```python
from build123d import *

# Parameters (mm, degrees)
ESQUISSE1_W             = 68
ESQUISSE1_H             = 1.6
EXTRUSION1_DEPTH        = 45
ESQUISSE2_W             = 25
ESQUISSE2_H             = 34
ENL_V_MAT_EXTRU_1_DEPTH = 2
ESQUISSE4_W             = 4.000005344
ESQUISSE4_H             = 8.5
ENL_V_MAT_EXTRU_2_DEPTH = 0.1
ESQUISSE5_W             = 4.000005344
ESQUISSE5_H             = 8.5
ENL_V_MAT_EXTRU_3_DEPTH = 0.1


with BuildPart() as part:
    # Esquisse1 → Extrusion1 (new body)
    with BuildSketch(Plane.XY):
        with Locations((57.011095297, 71.602293989)):
            Rectangle(ESQUISSE1_W, ESQUISSE1_H)
    extrude(amount=EXTRUSION1_DEPTH)

    # Esquisse2 → Enlèv. mat.-Extru.1 (cut)
    with BuildSketch(Plane(origin=(0, 72.402293989, 0), x_dir=(-1, 0, 0), z_dir=(0, 1, 0))):
        with Locations((-78.511095297, 47)):
            Rectangle(ESQUISSE2_W, ESQUISSE2_H)
    extrude(amount=-ENL_V_MAT_EXTRU_1_DEPTH, mode=Mode.SUBTRACT)

    # Esquisse4 → Enlèv. mat.-Extru.2 (cut)
    with BuildSketch(Plane(origin=(0, 72.402293989, 0), x_dir=(-1, 0, 0), z_dir=(0, 1, 0))):
        with Locations((-89.011092625, 4.25)):
            Rectangle(ESQUISSE4_W, ESQUISSE4_H)
        Polygon((-27.011089953, 8.5), (-27.011089953, 0), (-23.011095297, 0), (-23.029811449, 8.5), align=None)
        Polygon((-83.761089902, 23.952607164), (-71.261089902, 23.952607164), (-71.261089902, 29.947835896), (-83.761089902, 30.082433695), align=None)
    extrude(amount=-ENL_V_MAT_EXTRU_2_DEPTH, mode=Mode.SUBTRACT)

    # Esquisse5 → Enlèv. mat.-Extru.3 (cut)
    with BuildSketch(Plane.XZ.offset(-70.802293989)):
        Polygon((23.029811449, 8.5), (23.011095297, 0), (27.011089953, 0), (27.011089953, 8.5), align=None)
        with Locations((89.011092625, 4.25)):
            Rectangle(ESQUISSE5_W, ESQUISSE5_H)
    extrude(amount=-ENL_V_MAT_EXTRU_3_DEPTH, mode=Mode.SUBTRACT)


solid = part.part
```
Here's how the part is built. I have some questions about the finished solid (model axes, mm). A direction names the side the tool comes from. Round coordinates to 2 decimals unless told otherwise and drop trailing zeros. Write each loop counter-clockwise with the first axis right and the second up, starting at its lowest first coordinate (ties: lowest second). Pieces come first, ordered by that corner, then holes.
Q1. If we mould it in two halves opening along Z, with no side actions, what happens to faces 6 (the flat face through (78, 72.302, 27)), 7 (the flat face through (89, 72.302, 4)), 8 (the flat face through (57, 72, 0)), 9 (the flat face through (44, 72, 45))? For each: +Z half, -Z half, draft (parallel to the pull), parting line (faces both ways), or undercut.
Q2. Which directions (+Z, -Z, +X, -X, +Y, -Y) give clear straight access to the entire face, cutting with the end or side of a thin tool? Please do faces 1 (the flat face through (25, 72.302, 4)), 2 (the flat face through (89, 70.902, 4)), 3 (the flat face through (66.011, 72, 37)), 4 (the flat face through (25, 70.902, 4)), 5 (the flat face through (23.011, 72, 22)).
Q3. Will these pins go through, and if not, where does the flat tip stop? P1, Ø5, axis at x = 78, z = 25.5, coming from the +Y side; P2, Ø1.2, axis at x = 25.5, z = 6, coming from the +Y side; P3, Ø4.5, axis at x = 89.5, z = 4, coming from the -Y side.
Q4. If we section it at A-A on y = 71.4: Write out the boundary of the cut face in (x, z).
Q5. Please list where these lines run through material, in increasing order: probe 1 along Z at (x, y) = (86, 72.1); probe 2 along X at (y, z) = (71.6, 42.5).
Answer below:
1. face 6: undercut
1. face 7: draft
1. face 8: -Z half
1. face 9: +Z half
2. face 1: -Z, +Y
2. face 2: -Z, +X, -Y
2. face 3: +Z, +X, +Y, -Y
2. face 4: -Z, -Y
2. face 5: +Z, -Z, -X, +Y, -Y
3. P1: stops at y = 72.4
3. P2: stops at y = 72.3
3. P3: stops at y = 70.9
4. outline: (23.01, 0) - (91.01, 0) - (91.01, 30) - (66.01, 30) - (66.01, 45) - (23.01, 45) - close
5. probe 1: z = 0 to 30
5. probe 2: x = 23.01 to 66.01
